```python
from build123d import *

# Parameters (mm, degrees)
SALIENTE_EXTRUIR2_DEPTH = 8
CORTAR_EXTRUIR1_DEPTH   = 8
CROQUIS4_R              = 4
SALIENTE_EXTRUIR3_DEPTH = 13
CROQUIS5_W              = 11
CROQUIS5_H              = 133.016244933
CORTAR_EXTRUIR2_DEPTH   = 87
CROQUIS7_R              = 1.5
CORTAR_EXTRUIR3_DEPTH   = 87
CROQUIS8_R              = 3.25
CORTAR_EXTRUIR4_DEPTH   = 3


with BuildPart() as part:
    # Croquis1 → Saliente-Extruir2 (new body)
    with BuildSketch(Plane(origin=(0, 0, 0), x_dir=(1, 0, 0), z_dir=(0, 1, 0))):
        Polygon((0, 0), (0, 40), (20, 40), (20, -40), (0, -40), align=None)
    extrude(amount=SALIENTE_EXTRUIR2_DEPTH)

    # Croquis3 → Cortar-Extruir1 (cut)
    with BuildSketch(Plane(origin=(0, 8, 0), x_dir=(1, 0, 0), z_dir=(0, 1, 0))):
        with BuildLine():
            Line((20, 40), (0.615528128, 40))
            ThreePointArc((0.615528128, 40), (11.819805153, 31.819805153), (20, 20.615528128))
            Line((20, 20.615528128), (20, 40))
        make_face()
        with BuildLine():
            ThreePointArc((20, -20.615528128), (11.819805153, -31.819805153), (0.615528128, -40))
            Line((0.615528128, -40), (20, -40))
            Line((20, -40), (20, -20.615528128))
        make_face()
    extrude(amount=-CORTAR_EXTRUIR1_DEPTH, mode=Mode.SUBTRACT)

    # Croquis4 → Saliente-Extruir3 (add)
    with BuildSketch(Plane(origin=(0, 0, 0), x_dir=(0, 0, -1), z_dir=(1, 0, 0))):
        with BuildLine():
            Line((0, 0), (-30, 0))
            Line((-30, 0), (-30, 5.63250108))
            ThreePointArc((-30, 5.63250108), (-28.111788424, 14.115609005), (-22.803687993, 20.996926672))
            Line((-22.803687993, 20.996926672), (23.866202653, 59.88850221))
            ThreePointArc((23.866202653, 59.88850221), (28.203401142, 64.948074064), (30.637508796, 71.151756681))
            ThreePointArc((30.637508796, 71.151756681), (51.597737237, 93.799339931), (81.447972358, 85.975807058))
            ThreePointArc((81.447972358, 85.975807058), (87.123427128, 70.974483465), (79.953012113, 56.627510094))
            Line((79.953012113, 56.627510094), (37.196312007, 20.996926672))
            ThreePointArc((37.196312007, 20.996926672), (31.888211576, 14.115609005), (30, 5.63250108))
            Line((30, 5.63250108), (30, 0))
            Line((30, 0), (0, 0))
        make_face()
        with Locations(Location((65, 80, 0), (0, 0, 180))):
            Circle(CROQUIS4_R, mode=Mode.SUBTRACT)
    extrude(amount=SALIENTE_EXTRUIR3_DEPTH)

    # Croquis5 → Cortar-Extruir2 (cut)
    with BuildSketch(Plane(origin=(0, 95, 0), x_dir=(1, 0, 0), z_dir=(0, 1, 0))):
        with Locations((14.5, 20.641201652)):
            Rectangle(CROQUIS5_W, CROQUIS5_H)
    extrude(amount=-CORTAR_EXTRUIR2_DEPTH, mode=Mode.SUBTRACT)

    # Croquis7 → Cortar-Extruir3 (cut)
    with BuildSketch(Plane(origin=(0, 8, 0), x_dir=(1, 0, 0), z_dir=(0, 1, 0))):
        with Locations(Location((14.5, 14.481175371, 0), (0, 0, 270))):
            Circle(CROQUIS7_R)
        with Locations(Location((14.5, 0.070310316, 0), (0, 0, 270))):
            Circle(CROQUIS7_R)
        with Locations(Location((14.5, -14.410865055, 0), (0, 0, 270))):
            Circle(CROQUIS7_R)
    extrude(amount=-CORTAR_EXTRUIR3_DEPTH, mode=Mode.SUBTRACT)

    # Croquis8 → Cortar-Extruir4 (cut)
    with BuildSketch(Plane(origin=(0, 8, 0), x_dir=(1, 0, 0), z_dir=(0, 1, 0))):
        with Locations(Location((14.5, 14.481175371, 0), (0, 0, 270))):
            Circle(CROQUIS8_R)
        with Locations(Location((14.5, 0.070310316, 0), (0, 0, 270))):
            Circle(CROQUIS8_R)
        with Locations(Location((14.5, -14.410865055, 0), (0, 0, 270))):
            Circle(CROQUIS8_R)
    extrude(amount=-CORTAR_EXTRUIR4_DEPTH, mode=Mode.SUBTRACT)


solid = part.part
```
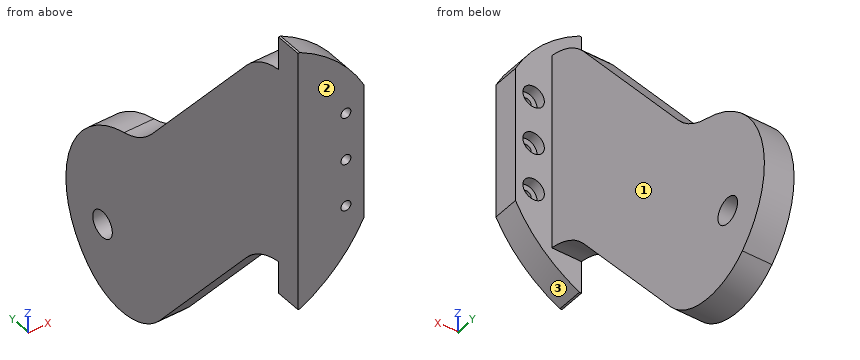
Part model, mm, in its own coordinate system. Face numbers are marked on the shaded views. A direction names the side the tool comes from. Give positions to 0.01 mm unless a question says otherwise; leave off trailing zeros. Order: outer loops, then holes, each group sorted by start corner. A loop starts at its lowest first (then second) coordinate and runs counter-clockwise, first axis right, second up. Notation, with made-up numbers: M 11,30.25 L 39,30.25 A24 ccw 39,52.25 Z; hole C 19,-7 d8. An arc over 180 degrees is marked long. Use a Markdown table: item, result. Add a question column.
(1) Probe line 1 along Y through (x, z) = (16.5, 26); line 2 along X through (y, z) = (65, -56.5); line 3 along Z through (x, y) = (2.5, 80). List the from-to ranges inside material, lowest first. Write a range as [from, to].
(2) 3-axis set-ups, long thin cutter, end or side, ignore diameter. For the marked faces 1, 2 and 3: which of +Z, -Z, +X, -X, +Y, -Y reach the whole face in a straight line?
(3) Drop flat-ended pins along their axis: P1, Ø3, axis at x = 13.5, z = 14, coming from the +Y side; P2, Ø10, axis at x = 5.5, z = 12.5, coming from the +Y side; P3, Ø7, axis at x = 16, z = -1, coming from the +Y side; P4, Ø8, axis at x = 16, z = -47.5, coming from the -Y side. Give the stop position or say it passes through.
(4) Saw through at C-C, the plane z = -65. Give the cut face in (x, y), and give its area (3 significant figures).
(5) Saw through at A-A, the plane x = 7. Give the cut face in (y, z), and give its area (3 significant figures).
(6) Saw through at D-D, the plane x = 14.5. Give the cut face in (y, z).
(7) Saw through at B-B, the plane y = 80. Give the cut face in (x, z).
Answer key:
| question | item | result |
|---|---|---|
| 1 | line 1 | [0, 8] |
| 1 | line 2 | [0, 9] |
| 1 | line 3 | [-85.48, -69], [-61, -34.02] |
| 2 | face 1 | +Z, -Z, +X, +Y |
| 2 | face 2 | +Z, -Z, +X, -X, -Y |
| 2 | face 3 | -Z, +X, -Y |
| 3 | P1 | y = 5 |
| 3 | P2 | y = 33.75 |
| 3 | P3 | y = 8 |
| 3 | P4 | through |
| 4 | outline | M 0,44.17 L 9,44.17 L 9,76 L 0,76 Z; M 0,84 L 9,84 L 9,94.58 L 0,94.58 Z |
| 4 | area | 382 mm^2 |
| 5 | outline | M 0,-36 L 8,-36 L 8,-30.14 A20 cw 21,-37.2 L 56.63,-79.95 A20 ccw 85.98,-81.45 A30 ccw 71.15,-30.64 A20 cw 59.89,-23.87 L 21,22.8 A20 ccw 8,29.86 L 8,36 L 0,36 Z; hole C 80,-65 d8 |
| 5 | area | 5,320 mm^2 |
| 6 | outline | M 0,-28.89 L 8,-28.89 L 8,-17.73 L 5,-17.73 L 5,-15.98 L 0,-15.98 Z; M 0,-12.98 L 5,-12.98 L 5,-11.23 L 8,-11.23 L 8,-3.32 L 5,-3.32 L 5,-1.57 L 0,-1.57 Z; M 0,1.43 L 5,1.43 L 5,3.18 L 8,3.18 L 8,11.16 L 5,11.16 L 5,12.91 L 0,12.91 Z; M 0,15.91 L 5,15.91 L 5,17.66 L 8,17.66 L 8,28.89 L 0,28.89 Z |
| 7 | outline | M 0,-85.48 L 9,-85.48 L 9,-69 L 0,-69 Z; M 0,-61 L 9,-61 L 9,-34.02 L 0,-34.02 Z |
